from build123d import *

# Parameters (mm, degrees)
SKETCH1_W               = 200
SKETCH1_H               = 200
BOSS_EXTRUDE1_DEPTH     = 20
BOSS_EXTRUDE2_DEPTH     = 20
SKETCH2_4_R             = 3.7970867
CUT_EXTRUDE2_DEPTH      = 10
MIRROR4_COPY_1_DEPTH    = 20
MIRROR4_COPY_2_SKETCH_R = 3.7970867
MIRROR4_COPY_2_DEPTH    = 10
SKETCH3_W               = 188
SKETCH3_H               = 188
CUT_EXTRUDE1_DEPTH      = 21


with BuildPart() as part:
    # Sketch1 → Boss-Extrude1 (new body)
    with BuildSketch(Plane(origin=(0, 0, 0), x_dir=(1, 0, 0), z_dir=(0, 1, 0))):
        with Locations((100, 100)):
            Rectangle(SKETCH1_W, SKETCH1_H)
    extrude(amount=BOSS_EXTRUDE1_DEPTH)

    # Sketch2 → Boss-Extrude2 (add)
    with BuildSketch(Plane.XZ):
        with BuildLine():
            Line((-17.087625271, 2.945489647), (0, -14.142135624))
            Line((0, -14.142135624), (0, 0))
            Line((0, 0), (14.142135624, 0))
            Line((14.142135624, 0), (-2.945489647, 17.087625271))
            ThreePointArc((-2.945489647, 17.087625271), (-17.087625271, 17.087625271), (-17.087625271, 2.945489647))
        make_face()
    boss_extrude2 = extrude(amount=-BOSS_EXTRUDE2_DEPTH)

    # Sketch2<4> → Cut-Extrude2 (cut)
    with BuildSketch(Plane.XZ):
        with Locations((-10.016557459, 10.016557459)):
            Circle(SKETCH2_4_R)
        with Locations((-3.415367361, 3.415367361)):
            Circle(SKETCH2_4_R)
    cut_extrude2 = extrude(amount=-CUT_EXTRUDE2_DEPTH, mode=Mode.SUBTRACT)

    # Mirror3: Boss-Extrude2, Cut-Extrude2 across plane
    add(boss_extrude2.mirror(Plane(origin=(100, 0, 0), x_dir=(0, 0, 1), z_dir=(1, 0, 0))))
    add(cut_extrude2.mirror(Plane(origin=(100, 0, 0), x_dir=(0, 0, 1), z_dir=(1, 0, 0))), mode=Mode.SUBTRACT)

    # Mirror4: Boss-Extrude2, Cut-Extrude2 across plane
    add(boss_extrude2.mirror(Plane(origin=(0, 0, -100), x_dir=(1, 0, 0), z_dir=(0, 0, -1))))
    add(cut_extrude2.mirror(Plane(origin=(0, 0, -100), x_dir=(1, 0, 0), z_dir=(0, 0, -1))), mode=Mode.SUBTRACT)

    # Mirror4 copy 1 sketch → Mirror4 copy 1 (add)
    with BuildSketch(Plane(origin=(200, 0, -200), x_dir=(-1, 0, 0), z_dir=(0, -1, 0))):
        with BuildLine():
            Line((-17.087625271, 2.945489647), (0, -14.142135624))
            Line((0, -14.142135624), (0, 0))
            Line((0, 0), (14.142135624, 0))
            Line((14.142135624, 0), (-2.945489647, 17.087625271))
            ThreePointArc((-2.945489647, 17.087625271), (-17.087625271, 17.087625271), (-17.087625271, 2.945489647))
        make_face()
    extrude(amount=-MIRROR4_COPY_1_DEPTH)

    # Mirror4 copy 2 sketch → Mirror4 copy 2 (cut)
    with BuildSketch(Plane(origin=(200, 0, -200), x_dir=(-1, 0, 0), z_dir=(0, -1, 0))):
        with Locations((-10.016557459, 10.016557459)):
            Circle(MIRROR4_COPY_2_SKETCH_R)
        with Locations((-3.415367361, 3.415367361)):
            Circle(MIRROR4_COPY_2_SKETCH_R)
    extrude(amount=-MIRROR4_COPY_2_DEPTH, mode=Mode.SUBTRACT)

    # Sketch3 → Cut-Extrude1 (cut, through all)
    with BuildSketch(Plane.XZ):
        with Locations((100, -100)):
            Rectangle(SKETCH3_W, SKETCH3_H)
    extrude(amount=-CUT_EXTRUDE1_DEPTH, mode=Mode.SUBTRACT)


solid = part.part
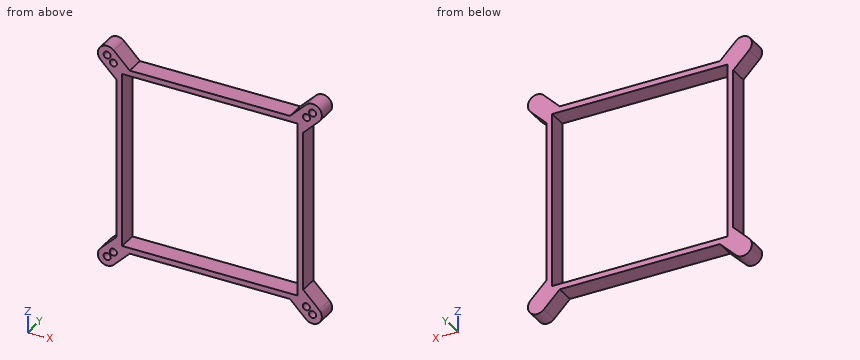
Verification items for the finished model (mm, model axes). Give positions to 0.01 mm unless a question says otherwise; leave off trailing zeros. Write each loop counter-clockwise with the first axis right and the second up, starting at its lowest first coordinate (ties: lowest second). Pieces come first, ordered by that corner, then holes. Notation, with made-up numbers: (60.25, 70.25) - (102.25, 70.25) arc R25 cw to (102.25, 88.25) - close; hole circle Ø9 at (31, 50.5). An arc over 180 degrees is marked (long way). Answer as CSV lines item,"result". Start each with the question number.
1. Depth check by flat-ended pin: pin 1 (6 mm diameter, centred on x = 71, y = 7.5, fed in from -Z); pin 2 (6 mm diameter, centred on y = 7.5, z = -73, fed in from -X); pin 3 (3 mm diameter, centred on y = 12, z = -172, fed in from +X). Enter the tip coordinate at first touch or a pass-through.
2. Sectioned sample at C-C (y = 16). Record the boundary of the cut face in (x, z).
3. Thickness scan on line 1 (Z direction, x = 140.5, y = 1); line 2 (X direction, y = 8.5, z = -45.5); line 3 (X direction, y = 4.75, z = -210). Record the ranges inside material, lowest first.
4. Sectioned sample at A-A (x = 99). Record the boundary of the cut face in (y, z).
5. Sectioned sample at B-B (z = -91.5). Record the boundary of the cut face in (x, y).
Derived:
1,pin 1,"z = -200"
1,pin 2,"x = 0"
1,pin 3,"x = 200"
2,outline,"(-17.09, -202.95) arc R10 ccw to (-2.95, -217.09) - (14.14, -200) - (185.86, -200) - (202.95, -217.09) arc R10 ccw to (217.09, -202.95) - (200, -185.86) - (200, -14.14) - (217.09, 2.95) arc R10 ccw to (202.95, 17.09) - (185.86, 0) - (14.14, 0) - (-2.95, 17.09) arc R10 ccw to (-17.09, 2.95) - (0, -14.14) - (0, -185.86) - close; hole (6, -194) - (194, -194) - (194, -6) - (6, -6) - close"
3,line 1,"-200 to -194, -6 to 0"
3,line 2,"0 to 6, 194 to 200"
3,line 3,"-20.02 to -13.81, -6.22 to 4.14, 195.86 to 206.22, 213.81 to 220.02"
4,outline,"(0, -200) - (20, -200) - (20, -194) - (0, -194) - close; (0, -6) - (20, -6) - (20, 0) - (0, 0) - close"
5,outline,"(0, 0) - (6, 0) - (6, 20) - (0, 20) - close; (194, 0) - (200, 0) - (200, 20) - (194, 20) - close"
